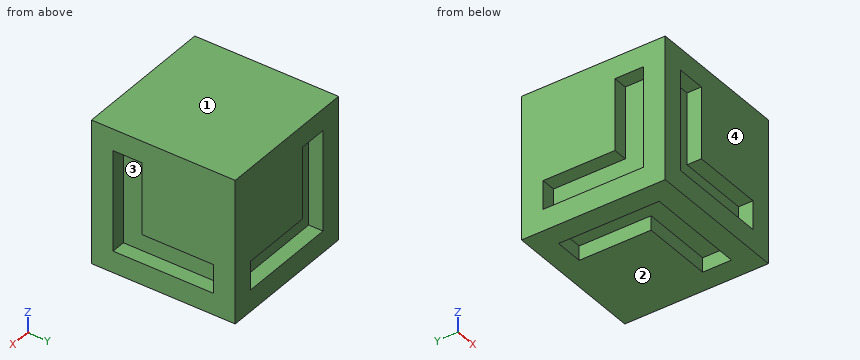
from build123d import *

# Parameters (mm, degrees)
SKETCH1_W           = 20
SKETCH1_H           = 20
BOSS_EXTRUDE1_DEPTH = 20
CUT_EXTRUDE1_DEPTH  = 2
CUT_EXTRUDE2_DEPTH  = 2
CUT_EXTRUDE3_DEPTH  = 2
CUT_EXTRUDE4_DEPTH  = 2
CUT_EXTRUDE5_DEPTH  = 2


with BuildPart() as part:
    # Sketch1 → Boss-Extrude1 (new body)
    with BuildSketch(Plane.XY.offset(5)):
        with Locations((20, 25)):
            Rectangle(SKETCH1_W, SKETCH1_H)
    extrude(amount=BOSS_EXTRUDE1_DEPTH)

    # Sketch2 → Cut-Extrude1 (cut)
    with BuildSketch(Plane(origin=(30, 0, 0), x_dir=(0, 0, -1), z_dir=(1, 0, 0))):
        Polygon((-8, 18), (-8, 32), (-12, 32), (-12, 22), (-22, 22), (-22, 18), align=None)
    extrude(amount=-CUT_EXTRUDE1_DEPTH, mode=Mode.SUBTRACT)

    # Sketch3 → Cut-Extrude2 (cut)
    with BuildSketch(Plane.ZY.offset(-10)):
        Polygon((8, 18), (8, 32), (12, 32), (12, 22), (22, 22), (22, 18), align=None)
    extrude(amount=-CUT_EXTRUDE2_DEPTH, mode=Mode.SUBTRACT)

    # Sketch4 → Cut-Extrude3 (cut)
    with BuildSketch(Plane(origin=(0, 35, 0), x_dir=(1, 0, 0), z_dir=(0, 1, 0))):
        Polygon((13, -8), (27, -8), (27, -12), (17, -12), (17, -22), (13, -22), align=None)
    extrude(amount=-CUT_EXTRUDE3_DEPTH, mode=Mode.SUBTRACT)

    # Sketch5 → Cut-Extrude4 (cut)
    with BuildSketch(Plane.XZ.offset(-15)):
        Polygon((13, 8), (27, 8), (27, 12), (17, 12), (17, 22), (13, 22), align=None)
    extrude(amount=-CUT_EXTRUDE4_DEPTH, mode=Mode.SUBTRACT)

    # Sketch6 → Cut-Extrude5 (cut)
    with BuildSketch(Plane(origin=(0, 0, 5), x_dir=(-1, 0, 0), z_dir=(0, 0, -1))):
        Polygon((-13, 18), (-27, 18), (-27, 22), (-17, 22), (-17, 32), (-13, 32), align=None)
    extrude(amount=-CUT_EXTRUDE5_DEPTH, mode=Mode.SUBTRACT)


solid = part.part
Build history of the part. All positions in model axes, mm. Face numbers are marked on the shaded views. Coordinates: 2 decimals unless noted, no trailing zeros. Order: outer loops, then holes, each group sorted by start corner. A loop starts at its lowest first (then second) coordinate and runs counter-clockwise, first axis right, second up. Notation, with made-up numbers: (-13.75, 42.25) - (1.25, 42.25) arc R26 cw to (1.25, 70.25) - close; hole circle Ø5 at (54.5, -8.75). An arc over 180 degrees is marked (long way). Write item = value, one per line. Start each with the question number.
1) Saw through at A-A on y = 19. Write the cut outline in (x, z).
2) Saw through at B-B on x = 25. Write the cut outline in (y, z).
3) Two-plate mould, pull along Z, no slides. Class the marked faces 1, 2, 3 and 4: pulls with the +Z half, pulls with the -Z half, needs draft (parallel to the pull), parting line crosses it, or undercut.
4) Flat gauge pin, fed straight in: pin 1 Ø8 at (x, z) = (14, 13.5) entering from +Y. Where does the tip first touch, or does it go through?
5) Saw through at C-C on z = 21.5. Write the cut outline in (x, y).
6) Wall check: line 1 along Y through (x, z) = (28.75, 8.5); line 2 along Y through (x, z) = (28.75, 16); line 3 along Z through (x, y) = (28.5, 22.25). Give the ranges that are in metal, low to high. Write a range as from..to.
7) Saw through at D-D on z = 10. Write the cut outline in (x, y), then the cut area to 3 significant figures.
From the geometry:
q1.outline = (10, 5) - (13, 5) - (13, 7) - (27, 7) - (27, 5) - (30, 5) - (30, 8) - (28, 8) - (28, 22) - (30, 22) - (30, 25) - (10, 25) - (10, 22) - (12, 22) - (12, 8) - (10, 8) - close
q2.outline = (15, 5) - (18, 5) - (18, 7) - (22, 7) - (22, 5) - (35, 5) - (35, 8) - (33, 8) - (33, 12) - (35, 12) - (35, 25) - (15, 25) - (15, 12) - (17, 12) - (17, 8) - (15, 8) - close
q3.face_1 = pulls with the +Z half
q3.face_2 = pulls with the -Z half
q3.face_3 = undercut
q3.face_4 = needs draft
q4.pin_1 = 35
q5.outline = (10, 15) - (13, 15) - (13, 17) - (17, 17) - (17, 15) - (30, 15) - (30, 18) - (28, 18) - (28, 22) - (30, 22) - (30, 35) - (17, 35) - (17, 33) - (13, 33) - (13, 35) - (10, 35) - (10, 22) - (12, 22) - (12, 18) - (10, 18) - close
q6.line_1 = 15..18, 32..35
q6.line_2 = 15..18, 22..35
q6.line_3 = 5..8, 12..25
q7.outline = (10, 15) - (13, 15) - (13, 17) - (27, 17) - (27, 15) - (30, 15) - (30, 18) - (28, 18) - (28, 32) - (30, 32) - (30, 35) - (27, 35) - (27, 33) - (13, 33) - (13, 35) - (10, 35) - (10, 32) - (12, 32) - (12, 18) - (10, 18) - close
q7.area = 288 mm^2
